Here's how the part is built. I have some questions about the finished solid (model axes, mm). A direction names the side the tool comes from. Round coordinates to 2 decimals unless told otherwise and drop trailing zeros. Order: outer loops, then holes, each group sorted by start corner. A loop starts at its lowest first (then second) coordinate and runs counter-clockwise, first axis right, second up.
Autodesk Inventor part; units mm, degrees
ref_plane "YZ Plane" through (0, 0, 0) normal (1, 0, 0) x (0, 1, 0)
ref_plane "XZ Plane" through (0, 0, 0) normal (0, 1, 0) x (-1, 0, 0)
ref_plane "XY Plane" through (0, 0, 0) normal (0, 0, 1) x (1, 0, 0)
ref_plane "Plano de trabalho1" through (0, 0, 0) normal (0, 0, 1) x (1, 0, 0)
sketch "Esboço1" plane through (0, 0, 0) normal (0, 0, 1) x (1, 0, 0)
  circle A0 centre (0, 0) radius 24
  circle A1 centre (0, 0) radius 23
  point P0 (0, 0)
  dimension "d0" = 1
extrude "Extrusão1" add sketch "Esboço1" against normal blind 5
sketch "Esboço2" plane through (0, 0, 0) normal (0, 0, 1) x (1, 0, 0)
  circle A0 centre (0, 0) radius 23
  circle A1 centre (0, 0) radius 25.5
  point P0 (0, 0)
  dimension "d3" = 2.5
extrude "Extrusão2" add sketch "Esboço2" along normal blind 7
sketch "Esboço3" plane through (0, 0, 7) normal (0, 0, 1) x (1, 0, 0)
  circle A0 centre (0, 0) radius 23
  point P0 (0, 0)
extrude "Extrusão3" add sketch "Esboço3" against normal blind 1
sketch "Esboço4" plane through (0, 0, 7) normal (0, 0, 1) x (1, 0, 0)
  circle A0 centre (0, 0) radius 11.5
  dimension "d8" = 23
extrude "Extrusão4" add sketch "Esboço4" along normal blind 27
sketch "Esboço5" plane through (0, 0, 34) normal (0, 0, 1) x (1, 0, 0)
  circle A0 centre (0, 0) radius 11.5
  circle A1 centre (0, 0) radius 10.5
  dimension "d11" = 1
extrude "Extrusão5" cut sketch "Esboço5" against normal through all contours A1
properties part number "Bocal de Saída"
1) If we section it at C-C (z = 27): Write out the boundary of the cut face in (x, y), plus the area to 3 significant figures.
2) For faces 4 (the cylindrical face through (-2.994, 22.804, 0.577)), 5 (the cylindrical face through (-1.5, -11.4, 20.3)), 6 (the cylindrical face through (10, 3.2, 20.2)), which set-ups out of +Z, -Z, +X, -X, +Y, -Y let a thin tool reach every point of the face, with its end or its side?
3) If we section it at D-D (y = 16): Write out the boundary of the cut face in (x, z), plus the area to 3 significant figures.
4) I need wall thicknesses on line 1 (Y direction, x = 0, z = -1); line 2 (Y direction, x = 0, z = 16.5); line 3 (Z direction, x = 3.5, y = -18.5). Which ranges of each line are inside material? Lowest first, please.
5) If we section it at A-A (x = 0): Write out the boundary of the cut face in (y, z), plus the area to 3 significant figures.
6) We'd pull the mould along X, two halves only. Please class faces 1 (the flat face through (15, -19, 0)), 2 (the flat face through (10, -5, 6)), 3 (the cylindrical face through (-23.977, 1.055, -2.465)): +X half, -X half, draft (parallel to the pull), parting line (faces both ways), or undercut.
7) I'm going to push flat-ended pins straight in: pin 1 (6 mm diameter, centred on y = 6.5, z = -1, fed in from +X); pin 2 (1.5 mm diameter, centred on y = 7, z = 5.5, fed in from -X); pin 3 (10 mm diameter, centred on x = 13, z = 26.5, fed in from +Y). Where does each tip first touch, or does it pass through?
Solutions:
1. outline: circle Ø23 at (0, 0); hole circle Ø21 at (0, 0)
1. area: 69.1 mm2
2. face 4: -Z
2. face 5: +Z
2. face 6: +Z, -Z
3. outline: (-19.86, 0) - (-17.89, 0) - (-17.89, -5) - (-16.52, -5) - (-16.52, 6) - (16.52, 6) - (16.52, -5) - (17.89, -5) - (17.89, 0) - (19.86, 0) - (19.86, 7) - (-19.86, 7) - close
3. area: 93.4 mm2
4. line 1: y = -24 to -23, 23 to 24
4. line 2: y = -11.5 to -10.5, 10.5 to 11.5
4. line 3: z = 6 to 7
5. outline: (-25.5, 0) - (-24, 0) - (-24, -5) - (-23, -5) - (-23, 6) - (-10.5, 6) - (-10.5, 34) - (-11.5, 34) - (-11.5, 7) - (-25.5, 7) - close; (10.5, 6) - (23, 6) - (23, -5) - (24, -5) - (24, 0) - (25.5, 0) - (25.5, 7) - (11.5, 7) - (11.5, 34) - (10.5, 34) - close
5. area: 124 mm2
6. face 1: draft
6. face 2: undercut
6. face 3: parting line
7. pin 1: stops at x = 25.23
7. pin 2: stops at x = -24.72
7. pin 3: stops at y = 8.26
